Part model, mm, in its own coordinate system. Face numbers are marked on the shaded views. A direction names the side the tool comes from. Coordinates: 2 decimals unless noted, no trailing zeros. Loops run counter-clockwise (first coordinate to the right, second up) from the corner with the lowest first, then second, coordinate; pieces in that order, holes last. Notation, with made-up numbers: (25.25, 30.5) -> (82.25, 30.5) arc R21 cw to (82.25, 37.5) -> close; hole circle Ø8 at (-34, -13.5). An arc over 180 degrees is marked (long way). Use one line per item in the form item = value. Start each with the question number.
(1) Pin check, flat tips, straight feed: P1, Ø0.7, axis at y = -0.5, z = -1.5, coming from the -X side; P2, Ø3.5, axis at x = 28.88, y = -5.99, coming from the +Z side; P3, Ø1.1, axis at x = 28, z = 2.5, coming from the -Y side; P4, Ø0.5, axis at x = 63.5, z = 1, coming from the -Y side. Stop position of each tip, or through.
(2) Band-saw the part on B-B on x = 33. Give the cut face in (y, z).
(3) 3-axis set-ups, long thin cutter, end or side, ignore diameter. For the marked faces 1, 2 and 3: which of +Z, -Z, +X, -X, +Y, -Y reach the whole face in a straight line?
(4) Band-saw the part on C-C on z = -2.5. Count the separate pieces of the cut face and the enclosed holes in it, then the cut area to 3 significant figures.
(5) Mould opens along Y. For the marked faces 4, 5 and 6 say: +Y half, -Y half, draft (parallel to the pull), parting line (faces both ways), or undercut.
(6) Drill centre lines: L1, parallel to Y at x = 50, z = -1.25; L2, parallel to Y at x = 54, z = -1.75; L3, parallel to Z at x = 49, y = -2.25. Where is each one in solid material? Low to high. Write a range as [from, to].
(7) Band-saw the part on A-A on x = 54. Give the cut face in (y, z).
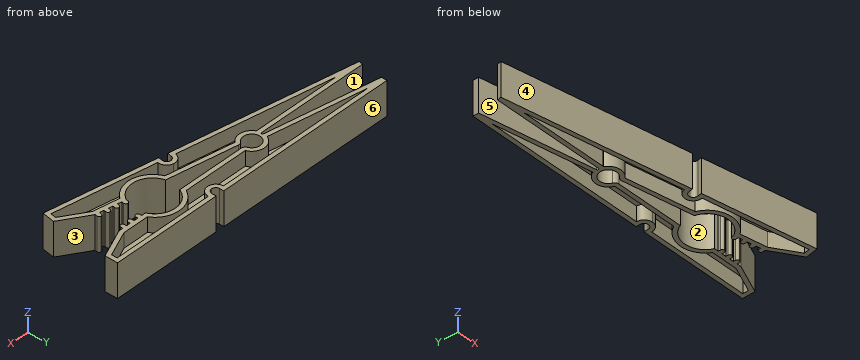
```python
from build123d import *

# Parameters (mm, degrees)
BRUTO_GRAMPO_1_START   = -4
BRUTO_GRAMPO_1_DEPTH   = 8
BRUTO_GRAMPO_1_START_2 = -0.5
BRUTO_GRAMPO_1_2_DEPTH = 1
ESCALA1_SCALE          = 1.015


# Read off the part's stored shape, not the designer's step: Bruto-Grampo-1
with BuildPart() as part:
    # Bruto-Grampo-1 outline → Bruto-Grampo-1 (new body)
    with BuildSketch(Plane.XY.offset(BRUTO_GRAMPO_1_START)):
        with BuildLine():
            Line((63, -6), (64, -6))
            Line((64, -6), (71, -3))
            Line((71, -3), (71, 0))
            Line((71, 0), (45, 0))
            Line((45, 0), (45, -1))
            ThreePointArc((45, -1), (44.707106781, -1.707106781), (44, -2))
            ThreePointArc((44, -2), (43.292893219, -1.707106781), (43, -1))
            Line((43, -1), (43, 0))
            Line((43, 0), (0, 0))
            Line((0, 0), (0, -1.335144068))
            Line((0, -1.335144068), (26.146588044, -5.84317649))
            ThreePointArc((26.146588044, -5.84317649), (26.311379183, -6.124884785), (26.061766048, -6.335144068))
            Line((26.061766048, -6.335144068), (-0.562908784, -6.335144068))
            Line((-0.562908784, -6.335144068), (-0.732815701, -7.320604184))
            Line((-0.732815701, -7.320604184), (41.641969276, -14.626601592))
            Line((41.641969276, -14.626601592), (41.811876193, -13.641141477))
            ThreePointArc((41.811876193, -13.641141477), (42.220653111, -12.99408053), (42.967243225, -12.825588277))
            ThreePointArc((42.967243225, -12.825588277), (43.614304172, -13.234365196), (43.782796424, -13.98095531))
            Line((43.782796424, -13.98095531), (43.612889508, -14.966415425))
            Line((43.612889508, -14.966415425), (69.234852518, -19.383995254))
            Line((69.234852518, -19.383995254), (69.744573267, -16.427614907))
            Line((69.744573267, -16.427614907), (63.356073202, -12.281886143))
            Line((63.356073202, -12.281886143), (63.44102666, -11.789156085))
            ThreePointArc((63.44102666, -11.789156085), (63.356780534, -11.415861028), (63.03325006, -11.211472569))
            ThreePointArc((63.03325006, -11.211472569), (62.659955003, -11.295718696), (62.455566544, -11.619249169))
            Line((62.455566544, -11.619249169), (62.370613086, -12.111979227))
            Line((62.370613086, -12.111979227), (61.38515297, -11.94207231))
            Line((61.38515297, -11.94207231), (61.470106428, -11.449342252))
            ThreePointArc((61.470106428, -11.449342252), (61.385860302, -11.076047195), (61.062329829, -10.871658736))
            ThreePointArc((61.062329829, -10.871658736), (60.689034772, -10.955904863), (60.484646313, -11.279435336))
            Line((60.484646313, -11.279435336), (60.399692854, -11.772165394))
            Line((60.399692854, -11.772165394), (59.414232739, -11.602258477))
            Line((59.414232739, -11.602258477), (59.499186197, -11.109528419))
            ThreePointArc((59.499186197, -11.109528419), (59.414940071, -10.736233362), (59.091409597, -10.531844903))
            ThreePointArc((59.091409597, -10.531844903), (58.71811454, -10.61609103), (58.513726081, -10.939621503))
            Line((58.513726081, -10.939621503), (58.428772623, -11.432351561))
            Line((58.428772623, -11.432351561), (57.443312507, -11.262444644))
            Line((57.443312507, -11.262444644), (57.528265965, -10.769714587))
            ThreePointArc((57.528265965, -10.769714587), (57.444019839, -10.39641953), (57.120489366, -10.19203107))
            ThreePointArc((57.120489366, -10.19203107), (56.747194309, -10.276277197), (56.54280585, -10.59980767))
            Line((56.54280585, -10.59980767), (56.457852391, -11.092537728))
            ThreePointArc((56.457852391, -11.092537728), (51.559018801, -13.393037449), (47.558931741, -9.747468492))
            Line((47.558931741, -9.747468492), (31.445619908, -6.969311252))
            ThreePointArc((31.445619908, -6.969311252), (30.937336598, -7.013760518), (30.517142023, -7.303180937))
            ThreePointArc((30.517142023, -7.303180937), (27.034098374, -5.632261947), (30.885618205, -5.333333319))
            ThreePointArc((30.885618205, -5.333333319), (31.251076976, -5.816496576), (31.828427251, -5.999999999))
            Line((31.828427251, -5.999999999), (48, -5.999999999))
            ThreePointArc((48, -5.999999999), (52.5, -2.993196129), (57, -6))
            Line((57, -6), (58, -6))
            Line((58, -6), (58, -6.5))
            ThreePointArc((58, -6.5), (58.146446609, -6.853553391), (58.5, -7))
            ThreePointArc((58.5, -7), (58.853553391, -6.853553391), (59, -6.5))
            Line((59, -6.5), (59, -6))
            Line((59, -6), (60, -6))
            Line((60, -6), (60, -6.5))
            ThreePointArc((60, -6.5), (60.146446609, -6.853553391), (60.5, -7))
            ThreePointArc((60.5, -7), (60.853553391, -6.853553391), (61, -6.5))
            Line((61, -6.5), (61, -6))
            Line((61, -6), (62, -6))
            Line((62, -6), (62, -6.5))
            ThreePointArc((62, -6.5), (62.146446609, -6.853553391), (62.5, -7))
            ThreePointArc((62.5, -7), (62.853553391, -6.853553391), (63, -6.5))
            Line((63, -6.5), (63, -6))
        make_face()
        with BuildLine():
            Line((68.419299318, -18.228628222), (44.76825654, -14.150862226))
            ThreePointArc((44.76825654, -14.150862226), (44.431272035, -12.657681998), (43.137150142, -11.840128162))
            ThreePointArc((43.137150142, -11.840128162), (41.643969914, -12.177112667), (40.826416077, -13.47123456))
            Line((40.826416077, -13.47123456), (5.237091217, -7.335144068))
            Line((5.237091217, -7.335144068), (26.061766048, -7.335144068))
            ThreePointArc((26.061766048, -7.335144068), (26.18246919, -7.329318154), (26.302050161, -7.311894575))
            ThreePointArc((26.302050161, -7.311894575), (28.615430589, -8.975249078), (31.27571299, -7.954771367))
            Line((31.27571299, -7.954771367), (46.78652147, -10.629048718))
            ThreePointArc((46.78652147, -10.629048718), (51.394904099, -14.37957122), (56.91703012, -12.186460714))
            Line((56.91703012, -12.186460714), (62.983893007, -13.232471556))
            Line((62.983893007, -13.232471556), (68.647077183, -16.907516604))
            Line((68.647077183, -16.907516604), (68.419299318, -18.228628222))
        make_face(mode=Mode.SUBTRACT)
        with BuildLine():
            ThreePointArc((31.828427251, -4.999999999), (29.084046667, -3.001177418), (26.232021768, -4.84315203))
            Line((26.232021768, -4.84315203), (3.941739992, -1))
            Line((3.941739992, -1), (42, -1))
            ThreePointArc((42, -1), (42.585786438, -2.414213562), (44, -3))
            ThreePointArc((44, -3), (45.414213562, -2.414213562), (46, -1))
            Line((46, -1), (70, -1))
            Line((70, -1), (70, -2.340603842))
            Line((70, -2.340603842), (63.794742298, -5))
            Line((63.794742298, -5), (57.624803191, -5))
            ThreePointArc((57.624803191, -5), (52.500000001, -1.993196129), (47.37519681, -4.999999999))
            Line((47.37519681, -4.999999999), (31.828427251, -4.999999999))
        make_face(mode=Mode.SUBTRACT)
    extrude(amount=BRUTO_GRAMPO_1_DEPTH)

    # Bruto-Grampo-1 2 outline → Bruto-Grampo-1 2 (add)
    with BuildSketch(Plane.XY.offset(BRUTO_GRAMPO_1_START_2)):
        with BuildLine():
            ThreePointArc((43.137150142, -11.840128162), (44.431272035, -12.657681998), (44.76825654, -14.150862226))
            Line((44.76825654, -14.150862226), (68.419299318, -18.228628222))
            Line((68.419299318, -18.228628222), (68.647077183, -16.907516604))
            Line((68.647077183, -16.907516604), (62.983893007, -13.232471556))
            Line((62.983893007, -13.232471556), (56.91703012, -12.186460714))
            ThreePointArc((56.91703012, -12.186460714), (51.394904099, -14.37957122), (46.78652147, -10.629048718))
            Line((46.78652147, -10.629048718), (31.27571299, -7.954771367))
            ThreePointArc((31.27571299, -7.954771367), (28.615430589, -8.975249078), (26.302050161, -7.311894575))
            ThreePointArc((26.302050161, -7.311894575), (26.18246919, -7.329318154), (26.061766048, -7.335144068))
            Line((26.061766048, -7.335144068), (5.237091217, -7.335144068))
            Line((5.237091217, -7.335144068), (40.826416077, -13.47123456))
            ThreePointArc((40.826416077, -13.47123456), (41.643969914, -12.177112667), (43.137150142, -11.840128162))
        make_face()
        with BuildLine():
            Line((3.941739992, -1), (26.232021768, -4.84315203))
            ThreePointArc((26.232021768, -4.84315203), (29.084046667, -3.001177418), (31.828427251, -4.999999999))
            Line((31.828427251, -4.999999999), (47.37519681, -4.999999999))
            ThreePointArc((47.37519681, -4.999999999), (52.500000001, -1.993196129), (57.624803191, -5))
            Line((57.624803191, -5), (63.794742298, -5))
            Line((63.794742298, -5), (70, -2.340603842))
            Line((70, -2.340603842), (70, -1))
            Line((70, -1), (46, -1))
            ThreePointArc((46, -1), (45.414213562, -2.414213562), (44, -3))
            ThreePointArc((44, -3), (42.585786438, -2.414213562), (42, -1))
            Line((42, -1), (3.941739992, -1))
        make_face()
    extrude(amount=BRUTO_GRAMPO_1_2_DEPTH)


with BuildPart() as part_1:
    # Escala1: scaled about (37.195426372, -6.887443952, 0)
    add(part.part.scale(ESCALA1_SCALE).moved(Location((-0.557931396, 0.103311659, 0))))


solid = part_1.part
```
A:
q1.P1 = -0.56
q1.P2 = through
q1.P3 = -12.47
q1.P4 = -18.54
q2.outline = (-13.24, -4.06) -> (-12.21, -4.06) -> (-12.21, -0.51) -> (-8.28, -0.51) -> (-8.28, -4.06) -> (-7.25, -4.06) -> (-7.25, 4.06) -> (-8.28, 4.06) -> (-8.28, 0.51) -> (-12.21, 0.51) -> (-12.21, 4.06) -> (-13.24, 4.06) -> close; (-5.99, -4.06) -> (-4.97, -4.06) -> (-4.97, -0.51) -> (-0.91, -0.51) -> (-0.91, -4.06) -> (0.1, -4.06) -> (0.1, 4.06) -> (-0.91, 4.06) -> (-0.91, 0.51) -> (-4.97, 0.51) -> (-4.97, 4.06) -> (-5.99, 4.06) -> close
q3.face_1 = +Z, -Z, -X
q3.face_2 = +Z, -Z
q3.face_3 = +Z, -Z, +X
q4.separate_pieces = 1
q4.enclosed_holes = 2
q4.area = 313 mm²
q5.face_4 = -Y half
q5.face_5 = undercut
q5.face_6 = +Y half
q6.L1 = [-16.17, -15.14], [-14.01, -12.86], [-3.76, -2.58], [-0.91, 0.1]
q6.L2 = [-16.86, -15.83], [-14.37, -13.32], [-3.1, -2.06], [-0.91, 0.1]
q6.L3 = [-0.51, 0.51]
q7.outline = (-16.86, -4.06) -> (-15.83, -4.06) -> (-15.83, -0.51) -> (-14.37, -0.51) -> (-14.37, -4.06) -> (-13.32, -4.06) -> (-13.32, 4.06) -> (-14.37, 4.06) -> (-14.37, 0.51) -> (-15.83, 0.51) -> (-15.83, 4.06) -> (-16.86, 4.06) -> close; (-3.1, -4.06) -> (-2.06, -4.06) -> (-2.06, -0.51) -> (-0.91, -0.51) -> (-0.91, -4.06) -> (0.1, -4.06) -> (0.1, 4.06) -> (-0.91, 4.06) -> (-0.91, 0.51) -> (-2.06, 0.51) -> (-2.06, 4.06) -> (-3.1, 4.06) -> close
